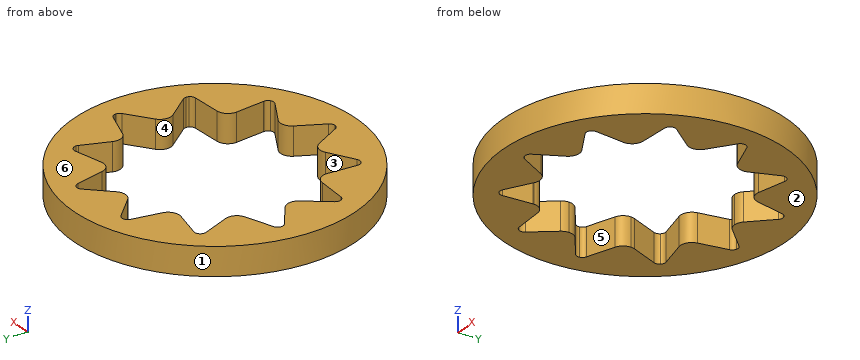
```python
from build123d import *

# Parameters (mm, degrees)
F0_R     = 15.875
F1_DEPTH = 3.175


with BuildPart() as f1:
    # F0 (on Top) → F1 (new body)
    with BuildSketch(Plane.XY):
        Circle(F0_R)
        with BuildLine():
            ThreePointArc((0, 13.49375), (1.920361, 13.356403), (3.801629, 12.947158))
            ThreePointArc((3.801629, 12.947158), (7.295272, 11.351665), (10.197896, 8.836527))
            ThreePointArc((10.197896, 8.836527), (12.274347, 5.605506), (13.356403, 1.920361))
            ThreePointArc((13.356403, 1.920361), (13.459369, 0.962633), (13.49375, 0))
            ThreePointArc((13.49375, 0), (13.185376, -2.868303), (12.274347, -5.605506))
            ThreePointArc((12.274347, -5.605506), (10.197896, -8.836527), (7.295272, -11.351665))
            ThreePointArc((7.295272, -11.351665), (3.801629, -12.947158), (0, -13.49375))
            ThreePointArc((0, -13.49375), (-3.801629, -12.947158), (-7.295272, -11.351665))
            ThreePointArc((-7.295272, -11.351665), (-10.197896, -8.836527), (-12.274347, -5.605506))
            ThreePointArc((-12.274347, -5.605506), (-13.356403, -1.920361), (-13.356403, 1.920361))
            ThreePointArc((-13.356403, 1.920361), (-12.274347, 5.605506), (-10.197896, 8.836527))
            ThreePointArc((-10.197896, 8.836527), (-7.295272, 11.351665), (-3.801629, 12.947158))
            ThreePointArc((-3.801629, 12.947158), (-1.920361, 13.356403), (0, 13.49375))
        make_face(mode=Mode.SUBTRACT)
        with BuildLine():
            ThreePointArc((-4.245319, 12.462805), (-4.090966, 12.766808), (-3.801629, 12.947158))
            ThreePointArc((-3.801629, 12.947158), (-7.295272, 11.351665), (-10.197896, 8.836527))
            ThreePointArc((-10.197896, 8.836527), (-9.913648, 9.024797), (-9.572997, 9.038914))
            Line((-9.572997, 9.038914), (-6.418023, 8.298951))
            ThreePointArc((-6.418023, 8.298951), (-6.916891, 10.530686), (-4.858029, 9.535398))
            ThreePointArc((-4.858029, 9.535398), (-4.864249, 9.409858), (-4.882848, 9.285548))
            Line((-4.882848, 9.285548), (-4.245319, 12.462805))
        make_face()
        with BuildLine():
            ThreePointArc((-6.418023, 8.298951), (-5.441415, 8.467007), (-4.882848, 9.285548))
            ThreePointArc((-4.882848, 9.285548), (-4.864249, 9.409858), (-4.858029, 9.535398))
            ThreePointArc((-4.858029, 9.535398), (-6.916891, 10.530686), (-6.418023, 8.298951))
        make_face()
        with BuildLine():
            ThreePointArc((-13.100136, 1.315559), (-13.312545, 1.58225), (-13.356403, 1.920361))
            ThreePointArc((-13.356403, 1.920361), (-13.356403, -1.920361), (-12.274347, -5.605506))
            ThreePointArc((-12.274347, -5.605506), (-12.327522, -5.268735), (-12.198852, -4.953004))
            Line((-12.198852, -4.953004), (-10.215134, -2.390531))
            ThreePointArc((-10.215134, -2.390531), (-12.476452, -1.793843), (-10.47484, -0.584239))
            Line((-10.47484, -0.584239), (-13.100136, 1.315559))
        make_face()
        with BuildLine():
            ThreePointArc((-9.949379, -1.613103), (-10.088347, -1.035463), (-10.47484, -0.584239))
            ThreePointArc((-10.47484, -0.584239), (-12.476452, -1.793843), (-10.215134, -2.390531))
            ThreePointArc((-10.215134, -2.390531), (-10.017653, -2.023901), (-9.949379, -1.613103))
        make_face()
        with BuildLine():
            ThreePointArc((-10.309291, 8.189186), (-10.343797, 8.528379), (-10.197896, 8.836527))
            ThreePointArc((-10.197896, 8.836527), (-12.274347, 5.605506), (-13.356403, 1.920361))
            ThreePointArc((-13.356403, 1.920361), (-13.219065, 2.232419), (-12.940124, 2.428465))
            Line((-12.940124, 2.428465), (-9.885936, 3.511676))
            ThreePointArc((-9.885936, 3.511676), (-11.465684, 5.236202), (-9.127859, 5.171633))
            Line((-9.127859, 5.171633), (-10.309291, 8.189186))
        make_face()
        with BuildLine():
            ThreePointArc((-9.040451, 4.708625), (-9.062495, 4.944219), (-9.127859, 5.171633))
            ThreePointArc((-9.127859, 5.171633), (-11.465684, 5.236202), (-9.885936, 3.511676))
            ThreePointArc((-9.885936, 3.511676), (-9.273139, 3.975902), (-9.040451, 4.708625))
        make_face()
        with BuildLine():
            Line((0, 12.60475), (0, 13.49375))
            ThreePointArc((0, 13.49375), (-1.920361, 13.356403), (-3.801629, 12.947158))
            ThreePointArc((-3.801629, 12.947158), (-3.460718, 12.951865), (-3.166512, 12.779572))
            Line((-3.166512, 12.779572), (-0.912433, 10.451367))
            ThreePointArc((-0.912433, 10.451367), (-1.169358, 11.830231), (0, 12.60475))
        make_face()
        with BuildLine():
            ThreePointArc((1.27, 11.33475), (0.898026, 12.232776), (0, 12.60475))
            Line((0, 12.60475), (0, 10.06475))
            ThreePointArc((0, 10.06475), (0.495481, 10.165392), (0.912433, 10.451367))
            ThreePointArc((0.912433, 10.451367), (1.177219, 10.858247), (1.27, 11.33475))
        make_face()
        with BuildLine():
            ThreePointArc((3.166512, 12.779572), (3.460718, 12.951865), (3.801629, 12.947158))
            ThreePointArc((3.801629, 12.947158), (1.920361, 13.356403), (0, 13.49375))
            Line((0, 13.49375), (0, 12.60475))
            ThreePointArc((0, 12.60475), (0.898026, 12.232776), (1.27, 11.33475))
            ThreePointArc((1.27, 11.33475), (1.177219, 10.858247), (0.912433, 10.451367))
            Line((0.912433, 10.451367), (3.166512, 12.779572))
        make_face()
        with BuildLine():
            Line((0, 10.06475), (0, 12.60475))
            ThreePointArc((0, 12.60475), (-1.169358, 11.830231), (-0.912433, 10.451367))
            ThreePointArc((-0.912433, 10.451367), (-0.495481, 10.165392), (0, 10.06475))
        make_face()
        with BuildLine():
            ThreePointArc((10.197896, 8.836527), (7.295272, 11.351665), (3.801629, 12.947158))
            ThreePointArc((3.801629, 12.947158), (4.090966, 12.766808), (4.245319, 12.462805))
            Line((4.245319, 12.462805), (4.882848, 9.285548))
            ThreePointArc((4.882848, 9.285548), (6.002488, 10.799178), (7.398029, 9.535398))
            ThreePointArc((7.398029, 9.535398), (7.123316, 8.746536), (6.418023, 8.298951))
            Line((6.418023, 8.298951), (9.572997, 9.038914))
            ThreePointArc((9.572997, 9.038914), (9.913648, 9.024797), (10.197896, 8.836527))
        make_face()
        with BuildLine():
            ThreePointArc((7.398029, 9.535398), (6.002488, 10.799178), (4.882848, 9.285548))
            ThreePointArc((4.882848, 9.285548), (5.441415, 8.467006), (6.418023, 8.298951))
            ThreePointArc((6.418023, 8.298951), (7.123316, 8.746536), (7.398029, 9.535398))
        make_face()
        with BuildLine():
            ThreePointArc((13.356403, 1.920361), (12.274347, 5.605506), (10.197896, 8.836527))
            ThreePointArc((10.197896, 8.836527), (10.312958, 8.6426), (10.352995, 8.420691))
            ThreePointArc((10.352995, 8.420691), (10.341973, 8.302894), (10.309291, 8.189187))
            Line((10.309291, 8.189187), (9.127859, 5.171633))
            ThreePointArc((9.127859, 5.171633), (10.546044, 5.956582), (11.580451, 4.708625))
            ThreePointArc((11.580451, 4.708625), (11.043174, 3.671313), (9.885936, 3.511676))
            Line((9.885936, 3.511676), (12.940124, 2.428466))
            ThreePointArc((12.940124, 2.428466), (13.219065, 2.23242), (13.356403, 1.920361))
        make_face()
        with BuildLine():
            ThreePointArc((9.127859, 5.171633), (9.155219, 4.181048), (9.885936, 3.511676))
            ThreePointArc((9.885936, 3.511676), (11.043174, 3.671313), (11.580451, 4.708625))
            ThreePointArc((11.580451, 4.708625), (10.546044, 5.956582), (9.127859, 5.171633))
        make_face()
        with BuildLine():
            ThreePointArc((13.49375, 0), (13.459369, 0.962633), (13.356403, 1.920361))
            ThreePointArc((13.356403, 1.920361), (13.361249, 1.875291), (13.362866, 1.829991))
            ThreePointArc((13.362866, 1.829991), (13.293382, 1.541171), (13.100136, 1.315559))
            Line((13.100136, 1.315559), (10.47484, -0.584239))
            ThreePointArc((10.47484, -0.584239), (11.797019, -0.482072), (12.489379, -1.613103))
            ThreePointArc((12.489379, -1.613103), (11.630177, -2.814829), (10.215134, -2.390531))
            Line((10.215134, -2.390531), (12.198853, -4.953004))
            ThreePointArc((12.198853, -4.953004), (12.297593, -5.136319), (12.33173, -5.341718))
            ThreePointArc((12.33173, -5.341718), (12.317219, -5.476697), (12.274347, -5.605506))
            ThreePointArc((12.274347, -5.605506), (13.185376, -2.868303), (13.49375, 0))
        make_face()
        with BuildLine():
            ThreePointArc((12.489379, -1.613103), (11.797019, -0.482072), (10.47484, -0.584239))
            ThreePointArc((10.47484, -0.584239), (9.962305, -1.432363), (10.215134, -2.390531))
            ThreePointArc((10.215134, -2.390531), (11.630177, -2.814829), (12.489379, -1.613103))
        make_face()
        with BuildLine():
            ThreePointArc((7.295272, -11.351665), (10.197896, -8.836527), (12.274347, -5.605506))
            ThreePointArc((12.274347, -5.605506), (12.054655, -5.866232), (11.73178, -5.97575))
            Line((11.73178, -5.97575), (8.496133, -6.154619))
            ThreePointArc((8.496133, -6.154619), (9.439122, -6.500206), (9.836232, -7.422683))
            ThreePointArc((9.836232, -7.422683), (8.621825, -8.691465), (7.301099, -7.533761))
            Line((7.301099, -7.533761), (7.584532, -10.76193))
            ThreePointArc((7.584532, -10.76193), (7.586357, -10.789673), (7.586965, -10.817469))
            ThreePointArc((7.586965, -10.817469), (7.509291, -11.121792), (7.295272, -11.351665))
        make_face()
        with BuildLine():
            ThreePointArc((9.836232, -7.422683), (9.439122, -6.500206), (8.496133, -6.154619))
            ThreePointArc((8.496133, -6.154619), (7.606431, -6.59101), (7.301099, -7.533761))
            ThreePointArc((7.301099, -7.533761), (8.621825, -8.691465), (9.836232, -7.422683))
        make_face()
        with BuildLine():
            ThreePointArc((0, -13.49375), (3.801629, -12.947158), (7.295272, -11.351665))
            ThreePointArc((7.295272, -11.351665), (6.969497, -11.452227), (6.638667, -11.3698))
            Line((6.638667, -11.3698), (3.819964, -9.770951))
            ThreePointArc((3.819964, -9.770951), (4.290792, -10.236425), (4.463368, -10.875613))
            ThreePointArc((4.463368, -10.875613), (2.889251, -12.108663), (2.069017, -10.285075))
            Line((2.069017, -10.285075), (0.562176, -13.154019))
            ThreePointArc((0.562176, -13.154019), (0.328428, -13.402221), (0, -13.49375))
        make_face()
        with BuildLine():
            ThreePointArc((4.463368, -10.875613), (4.290792, -10.236425), (3.819964, -9.770951))
            ThreePointArc((3.819964, -9.770951), (2.835568, -9.657057), (2.069017, -10.285075))
            ThreePointArc((2.069017, -10.285075), (2.889251, -12.108663), (4.463368, -10.875613))
        make_face()
        with BuildLine():
            ThreePointArc((-6.638667, -11.3698), (-6.969497, -11.452227), (-7.295272, -11.351665))
            ThreePointArc((-7.295272, -11.351665), (-3.801629, -12.947158), (0, -13.49375))
            ThreePointArc((0, -13.49375), (-0.328427, -13.402221), (-0.562175, -13.154019))
            Line((-0.562175, -13.154019), (-2.069017, -10.285075))
            ThreePointArc((-2.069017, -10.285075), (-1.960318, -10.571496), (-1.923368, -10.875613))
            ThreePointArc((-1.923368, -10.875613), (-3.832556, -11.973036), (-3.819964, -9.770951))
            Line((-3.819964, -9.770951), (-6.638667, -11.3698))
        make_face()
        with BuildLine():
            ThreePointArc((-2.069017, -10.285075), (-2.835568, -9.657057), (-3.819964, -9.770951))
            ThreePointArc((-3.819964, -9.770951), (-3.832556, -11.973036), (-1.923368, -10.875613))
            ThreePointArc((-1.923368, -10.875613), (-1.960318, -10.571496), (-2.069017, -10.285075))
        make_face()
        with BuildLine():
            ThreePointArc((-11.73178, -5.97575), (-12.054655, -5.866232), (-12.274347, -5.605506))
            ThreePointArc((-12.274347, -5.605506), (-10.197896, -8.836527), (-7.295272, -11.351665))
            ThreePointArc((-7.295272, -11.351665), (-7.522078, -11.097104), (-7.584532, -10.76193))
            Line((-7.584532, -10.76193), (-7.301099, -7.533761))
            ThreePointArc((-7.301099, -7.533761), (-9.526034, -8.254356), (-8.496133, -6.154619))
            Line((-8.496133, -6.154619), (-11.73178, -5.97575))
        make_face()
        with BuildLine():
            ThreePointArc((-7.296232, -7.422683), (-7.643756, -6.549793), (-8.496133, -6.154619))
            ThreePointArc((-8.496133, -6.154619), (-9.526034, -8.254356), (-7.301099, -7.533761))
            ThreePointArc((-7.301099, -7.533761), (-7.29745, -7.478275), (-7.296232, -7.422683))
        make_face()
    extrude(amount=-F1_DEPTH)


solid = f1.part
```
Input: part model. Units: mm. Frame: model coordinates. Face numbers are marked on the shaded views. A direction names the side the tool comes from. Coordinates: 2 decimals unless noted, no trailing zeros. Loops run counter-clockwise (first coordinate to the right, second up) from the corner with the lowest first, then second, coordinate; pieces in that order, holes last.
Q1. Set-up query: the marked faces 5 and 6. Return all of +Z, -Z, +X, -X, +Y, -Y with unobstructed straight access to the full face (end or side cutting, diameter ignored); none if empty.
Results are:
face 5: +Z, -Z
face 6: +Z, +X, -X, +Y, -Y
Q2. Line query: line 1 along X through (y, z) = (-10, -0.25); line 2 along Y through (x, z) = (12, -1.95); line 3 along X through (y, z) = (12, -2.5). Output: solid intervals per line, ascending.
Results are:
line 1: x = -12.33 to -7.52, -4.22 to -2.27, 2.27 to 4.22, 7.52 to 12.33
line 2: y = -10.39 to -5.9, -4.7 to 0.52, 2.76 to 10.39
line 3: x = -10.39 to -4.34, -2.41 to 2.41, 4.34 to 10.39
Q3. Section A-A, the plane y = -3. Return the cut outline in (x, z) (3 decimals).
Results are:
outline: (-15.589, -3.175) - (-10.687, -3.175) - (-10.687, 0) - (-15.589, 0) - close; (10.687, -3.175) - (15.589, -3.175) - (15.589, 0) - (10.687, 0) - close
Q4. Mould query, pull axis X, two halves, no side actions, for the marked faces 1, 2, 3 and 4. Classes: +X half, -X half, draft (parallel to the pull), parting line (faces both ways), or undercut.
Results are:
face 1: parting line
face 2: draft
face 3: undercut
face 4: undercut
Q5. Section B-B, the plane y = 11.5. Return the cut outline in (x, z) (1 decimal).
Results are:
outline: (-10.9, -3.2) - (-4.4, -3.2) - (-4.4, 0) - (-10.9, 0) - close; (-1.9, -3.2) - (1.9, -3.2) - (1.9, 0) - (-1.9, 0) - close; (4.4, -3.2) - (10.9, -3.2) - (10.9, 0) - (4.4, 0) - close
Q6. Contact query for a flat-ended pin moving along its axis: pin 1 (10 mm diameter, centred on x = -9.5, y = -5.5, fed in from +Z). Output: stop coordinate, or through.
Results are:
pin 1: stops at z = 0
